Check sheet for the drawn part. Datum: minimum x, y, z corner. Units: mm. A direction names the side the tool comes from. Coordinates: 2 decimals unless noted, no trailing zeros. Order: outer loops, then holes, each group sorted by start corner. A loop starts at its lowest first (then second) coordinate and runs counter-clockwise, first axis right, second up.
1. Draft check along X on the marked faces 1, 2, 3 and 4. Enter one of: released by +X, released by -X, zero draft, split by the parting line, or undercut.
2. Set-up check for the marked faces 5 and 6: record each of +Z, -Z, +X, -X, +Y, -Y from which the full face is reachable in a straight line by a thin tool's end or side.
3. Cross-section at D-D (y = 17.5). Enter the section's corners in (x, z).
4. Cross-section at A-A (z = 18). Enter the section's corners in (x, y).
5. Gauge pin test, flat ends, axial feed: pin 1 Ø1.2 at (y, z) = (30, 18) entering from -X; pin 2 Ø1.7 at (y, z) = (17.5, 30.5) entering from -X; pin 3 Ø1 at (x, y) = (50, 31) entering from -Z. Record the tip position at first contact, or that the pin passes through.
6. Cross-section at C-C (z = 30.5). Enter the section's corners in (x, y).
7. Thickness scan on line 1 (Y direction, x = 1.3, z = 18); line 2 (X direction, y = 6.5, z = 5.5); line 3 (Z direction, x = 56, y = 27.5). Record the ranges inside material, lowest first.
8. Cross-section at B-B (y = 30). Enter the section's corners in (x, z).
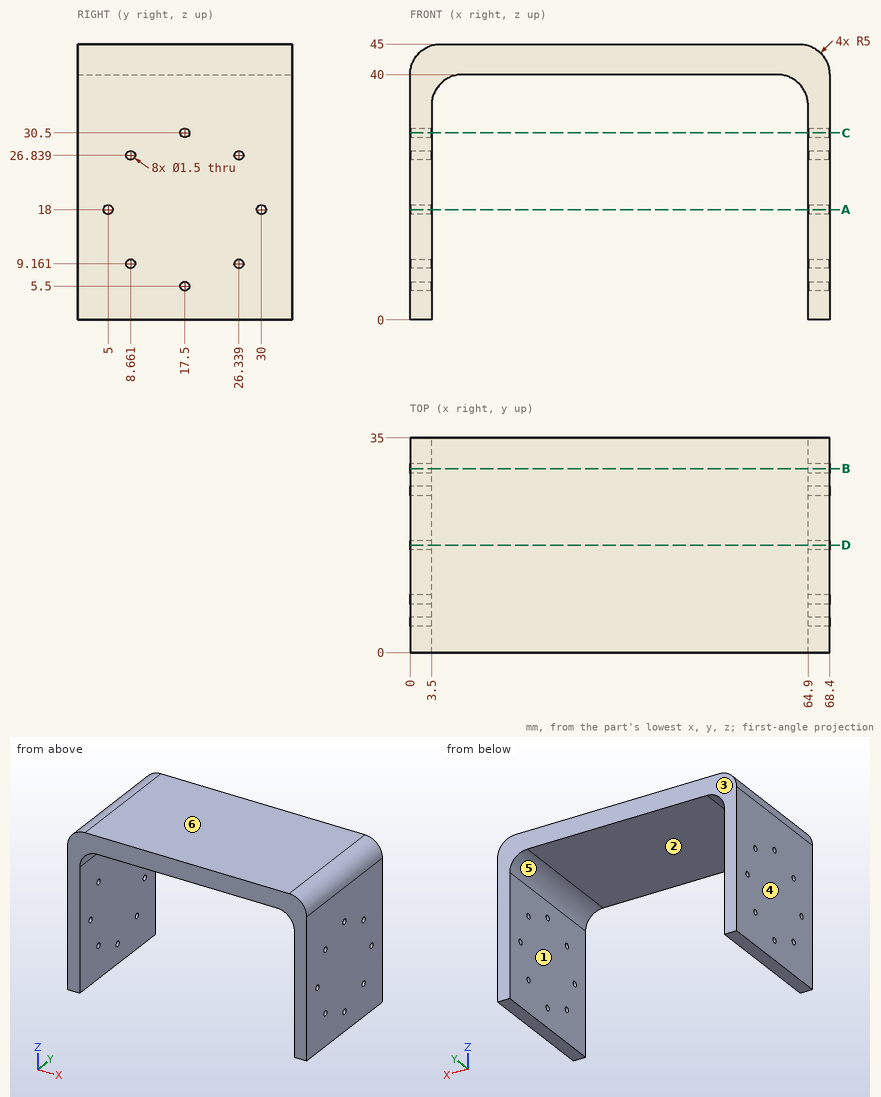
Data:
1. face 1: undercut
1. face 2: undercut
1. face 3: zero draft
1. face 4: released by -X
2. face 5: -Z, +Y, -Y
2. face 6: +Z, +X, -X, +Y, -Y
3. outline: (0, 0) - (3.5, 0) - (3.5, 4.75) - (0, 4.75) - close; (0, 6.25) - (3.5, 6.25) - (3.5, 29.75) - (0, 29.75) - close; (0, 31.25) - (3.5, 31.25) - (3.5, 35) arc R5 cw to (8.5, 40) - (59.9, 40) arc R5 cw to (64.9, 35) - (64.9, 31.25) - (68.4, 31.25) - (68.4, 40) arc R5 ccw to (63.4, 45) - (5, 45) arc R5 ccw to (0, 40) - close; (64.9, 0) - (68.4, 0) - (68.4, 4.75) - (64.9, 4.75) - close; (64.9, 6.25) - (68.4, 6.25) - (68.4, 29.75) - (64.9, 29.75) - close
4. outline: (0, 0) - (3.5, 0) - (3.5, 4.25) - (0, 4.25) - close; (0, 5.75) - (3.5, 5.75) - (3.5, 29.25) - (0, 29.25) - close; (0, 30.75) - (3.5, 30.75) - (3.5, 35) - (0, 35) - close; (64.9, 0) - (68.4, 0) - (68.4, 4.25) - (64.9, 4.25) - close; (64.9, 5.75) - (68.4, 5.75) - (68.4, 29.25) - (64.9, 29.25) - close; (64.9, 30.75) - (68.4, 30.75) - (68.4, 35) - (64.9, 35) - close
5. pin 1: passes through
5. pin 2: stops at x = 0
5. pin 3: stops at z = 40
6. outline: (0, 0) - (3.5, 0) - (3.5, 16.75) - (0, 16.75) - close; (0, 18.25) - (3.5, 18.25) - (3.5, 35) - (0, 35) - close; (64.9, 0) - (68.4, 0) - (68.4, 16.75) - (64.9, 16.75) - close; (64.9, 18.25) - (68.4, 18.25) - (68.4, 35) - (64.9, 35) - close
7. line 1: y = 0 to 4.25, 5.75 to 29.25, 30.75 to 35
7. line 2: x = 0 to 3.5, 64.9 to 68.4
7. line 3: z = 40 to 45
8. outline: (0, 0) - (3.5, 0) - (3.5, 17.25) - (0, 17.25) - close; (0, 18.75) - (3.5, 18.75) - (3.5, 35) arc R5 cw to (8.5, 40) - (59.9, 40) arc R5 cw to (64.9, 35) - (64.9, 18.75) - (68.4, 18.75) - (68.4, 40) arc R5 ccw to (63.4, 45) - (5, 45) arc R5 ccw to (0, 40) - close; (64.9, 0) - (68.4, 0) - (68.4, 17.25) - (64.9, 17.25) - close
